from build123d import *

# Parameters (mm, degrees)
SKETCH_1_W               = 60
SKETCH_1_H               = 32
EXTRUDE_1_DEPTH          = 3
SKETCH_3_R               = 36.5
EXTRUDE_2_DEPTH          = 2
SKETCH_4_R               = 1
CUT_EXTRUDE_2_DEPTH      = 10
PATTERN_CIRCULAR_1_COUNT = 8
SKETCH_5_R               = 5
CUT_EXTRUDE_3_DEPTH      = 3
SKETCH_6_R               = 3
EXTRUDE_3_DEPTH          = 5
SKETCH_7_R               = 1.62
CUT_EXTRUDE_4_DEPTH      = 5
SKETCH_9_R               = 2.6
CUT_EXTRUDE_5_DEPTH      = 2
SKETCH_10_R              = 20
EXTRUDE_4_DEPTH          = 3
SKETCH_11_R              = 1.25
CUT_EXTRUDE_6_DEPTH      = 10
PATTERN_CIRCULAR_2_COUNT = 4
SKETCH_12_W              = 42.513020476
SKETCH_12_H              = 32
CUT_EXTRUDE_7_DEPTH      = 3
SKETCH_13_R              = 6
CUT_EXTRUDE_8_DEPTH      = 10


with BuildPart() as part:
    # 草图1 → 凸台-拉伸1 (new body)
    with BuildSketch(Plane.XY):
        with Locations((-44.89426993, 6.0842078)):
            Rectangle(SKETCH_1_W, SKETCH_1_H)
    extrude(amount=EXTRUDE_1_DEPTH)

    # 草图3 → 凸台-拉伸2 (add)
    with BuildSketch(Plane.XY.offset(3)):
        with Locations((-44.89426993, 6.0842078)):
            Circle(SKETCH_3_R)
    extrude(amount=EXTRUDE_2_DEPTH)

    # 草图4 → 切除-拉伸2 (cut)
    with BuildSketch(Plane.XY.offset(5)):
        with Locations((-44.89426993, 29.0842078)):
            Circle(SKETCH_4_R)
    cut_extrude_2 = extrude(amount=-CUT_EXTRUDE_2_DEPTH, mode=Mode.SUBTRACT)

    # 阵列(圆周)1: 切除-拉伸2 ×8 about axis
    pattern_circular_1_axis = Axis((-44.89426993, 6.0842078, 0), (0, 0, 1))
    for i in range(1, PATTERN_CIRCULAR_1_COUNT):
        add(cut_extrude_2.rotate(pattern_circular_1_axis, i * 360 / PATTERN_CIRCULAR_1_COUNT), mode=Mode.SUBTRACT)

    # 草图5 → 切除-拉伸3 (cut)
    with BuildSketch(Plane(origin=(0, 0, 0), x_dir=(-1, 0, 0), z_dir=(0, 0, -1))):
        with Locations((28.630813963, 22.347663767)):
            Circle(SKETCH_5_R)
        with Locations((61.157725897, 22.347663767)):
            Circle(SKETCH_5_R)
        with Locations((28.630813963, -10.179248167)):
            Circle(SKETCH_5_R)
        with Locations((61.157725897, -10.179248167)):
            Circle(SKETCH_5_R)
    extrude(amount=-CUT_EXTRUDE_3_DEPTH, mode=Mode.SUBTRACT)

    # 草图6 → 凸台-拉伸3 (add)
    with BuildSketch(Plane(origin=(0, 0, 0), x_dir=(-1, 0, 0), z_dir=(0, 0, -1))):
        with Locations((21.89426993, 6.0842078)):
            Circle(SKETCH_6_R)
        with Locations((67.89426993, 6.0842078)):
            Circle(SKETCH_6_R)
    extrude(amount=-EXTRUDE_3_DEPTH)

    # 草图7 → 切除-拉伸4 (cut)
    with BuildSketch(Plane(origin=(0, 0, 0), x_dir=(-1, 0, 0), z_dir=(0, 0, -1))):
        with Locations((19.89426993, 12.0842078)):
            Circle(SKETCH_7_R)
        with Locations((19.89426993, 0.0842078)):
            Circle(SKETCH_7_R)
        with Locations((69.89426993, 12.0842078)):
            Circle(SKETCH_7_R)
        with Locations((69.89426993, 0.0842078)):
            Circle(SKETCH_7_R)
    extrude(amount=-CUT_EXTRUDE_4_DEPTH, mode=Mode.SUBTRACT)

    # 草图9 → 切除-拉伸5 (cut)
    with BuildSketch(Plane.XY.offset(5)):
        with Locations((-69.89426993, 12.0842078)):
            Circle(SKETCH_9_R)
        with Locations((-69.89426993, 0.0842078)):
            Circle(SKETCH_9_R)
        with Locations((-19.89426993, 12.0842078)):
            Circle(SKETCH_9_R)
        with Locations((-19.89426993, 0.0842078)):
            Circle(SKETCH_9_R)
    extrude(amount=-CUT_EXTRUDE_5_DEPTH, mode=Mode.SUBTRACT)

    # 草图10 → 凸台-拉伸4 (add)
    with BuildSketch(Plane.XY.offset(5)):
        with Locations((-44.89426993, 6.0842078)):
            Circle(SKETCH_10_R)
    extrude(amount=EXTRUDE_4_DEPTH)

    # 草图11 → 切除-拉伸6 (cut)
    with BuildSketch(Plane.XY.offset(8)):
        with Locations((-44.89426993, 14.0842078)):
            Circle(SKETCH_11_R)
    cut_extrude_6 = extrude(amount=-CUT_EXTRUDE_6_DEPTH, mode=Mode.SUBTRACT)

    # 阵列(圆周)2: 切除-拉伸6 ×4 about axis
    pattern_circular_2_axis = Axis((-44.89426993, 6.0842078, 0), (0, 0, 1))
    for i in range(1, PATTERN_CIRCULAR_2_COUNT):
        add(cut_extrude_6.rotate(pattern_circular_2_axis, i * 360 / PATTERN_CIRCULAR_2_COUNT), mode=Mode.SUBTRACT)

    # 草图12 → 切除-拉伸7 (cut)
    with BuildSketch(Plane(origin=(0, 0, 0), x_dir=(-1, 0, 0), z_dir=(0, 0, -1))):
        with Locations((44.89426993, 6.0842078)):
            Rectangle(SKETCH_12_W, SKETCH_12_H)
    extrude(amount=-CUT_EXTRUDE_7_DEPTH, mode=Mode.SUBTRACT)

    # 草图13 → 切除-拉伸8 (cut)
    with BuildSketch(Plane.XY.offset(8)):
        with Locations((-44.89426993, 6.0842078)):
            Circle(SKETCH_13_R)
    extrude(amount=-CUT_EXTRUDE_8_DEPTH, mode=Mode.SUBTRACT)


solid = part.part
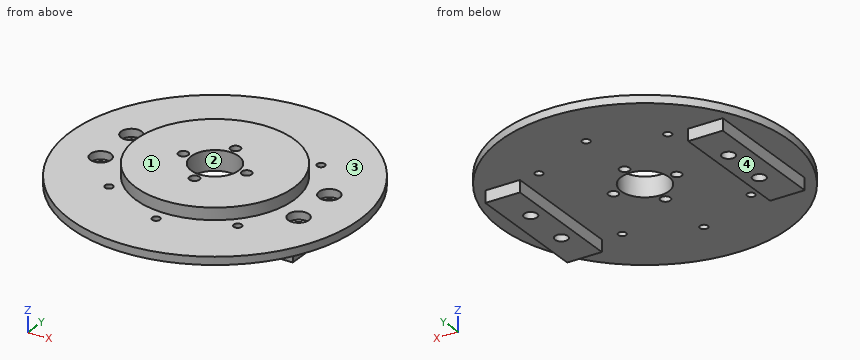
The model under review builds one solid part; all positions refer to its coordinate system, in mm. Face numbers are marked on the shaded views. A direction names the side the tool comes from. Round coordinates to 2 decimals unless told otherwise and drop trailing zeros. Order: outer loops, then holes, each group sorted by start corner. A loop starts at its lowest first (then second) coordinate and runs counter-clockwise, first axis right, second up. Notation, with made-up numbers: (58.25, 48.5) -> (78.25, 48.5) arc R15 ccw to (78.25, 68.5) -> close; hole circle Ø4 at (11.5, 59.25). An arc over 180 degrees is marked (long way). Return JSON: item names as keys, results as strings.
1. Take a section at B-B (x = -20). Write out the cut boundary in (y, z), then the cut area to 3 significant figures.
Answer block:
{"outline": "(-20.61, 3) -> (-9.92, 3) -> (-9.92, 0) -> (-1.53, 0) -> (-1.53, 3) -> (-2.51, 3) -> (-2.51, 5) -> (-20.61, 5) -> close; (1.7, 0) -> (10.47, 0) -> (10.47, 3) -> (9.49, 3) -> (9.49, 5) -> (2.68, 5) -> (2.68, 3) -> (1.7, 3) -> close; (13.7, 0) -> (22.08, 0) -> (22.08, 3) -> (32.78, 3) -> (32.78, 5) -> (14.68, 5) -> (14.68, 3) -> (13.7, 3) -> close", "area": "163 mm²"}
2. Take a section at D-D (y = -4). Write out the cut boundary in (x, z).
Answer block:
{"outline": "(-79.97, 3) -> (-74.89, 3) -> (-74.89, 0) -> (-66.15, 0) -> (-66.15, 3) -> (-23.64, 3) -> (-23.64, 0) -> (-14.89, 0) -> (-14.89, 3) -> (-9.81, 3) -> (-9.81, 5) -> (-27.62, 5) -> (-27.62, 8) -> (-62.17, 8) -> (-62.17, 5) -> (-79.97, 5) -> close"}
3. For L1, parallel to X at y = -2, z = 2; L2, parallel to Z at x = -33, y = 10.5; L3, parallel to Z at x = -65, y = 33.5, list the stretches that pass through material, from the lowest coordinate up. Write a range as [from, to].
Answer block:
{"L1": "x = [-74.89, -66.15], [-23.64, -14.89]", "L2": "z = [3, 8]", "L3": "z = [3, 5]"}
4. Take a section at C-C (x = -48). Write out the cut boundary in (y, z), then the cut area to 3 significant figures.
Answer block:
{"outline": "(-30.28, 3) -> (0.95, 3) -> (0.95, 8) -> (-13.67, 8) -> (-13.67, 5) -> (-30.28, 5) -> close; (11.22, 3) -> (42.45, 3) -> (42.45, 5) -> (25.84, 5) -> (25.84, 8) -> (11.22, 8) -> close", "area": "213 mm²"}
5. Insertion check: P1, Ø3, axis at x = -19.89, y = 0.08, coming from the -Z side; P2, Ø3.5, axis at x = -69, z = 2, coming from the -Y side; P3, Ø1.5, axis at x = -59.5, z = 4, coming from the +Y side; P4, Ø1.5, axis at y = 10.5, z = 3.5, coming from the -X side. Each pin has a flat end and moves straight along its axis. Give the tip position at first contact, or say it passes through.
Answer block:
{"P1": "passes through", "P2": "stops at y = -22.52", "P3": "stops at y = 39.85", "P4": "stops at x = -81.21"}
6. For the marked faces 3 and 4, list the 3-axis set-ups (+Z, -Z, +X, -X, +Y, -Y) from which the entire face can be reached by the end or side of a thin tool; tool diameter is ignored.
Answer block:
{"face 3": "+Z", "face 4": "-Z, +X, -X, +Y, -Y"}
7. The part is to be moulded in two halves that separate along Y. For the marked faces 1 and 2, say which applies: +Y half, -Y half, draft (parallel to the pull), parting line (faces both ways), or undercut.
Answer block:
{"face 1": "draft", "face 2": "undercut"}
8. Take a section at A-A (z = 1). Write out the cut boundary in (x, y).
Answer block:
{"outline": "(-74.89, -9.92) -> (-66.15, -9.92) -> (-66.15, 22.08) -> (-74.89, 22.08) -> close; (-23.64, -9.92) -> (-14.89, -9.92) -> (-14.89, 22.08) -> (-23.64, 22.08) -> close; hole circle Ø3.24 at (-69.89, 0.08); hole circle Ø3.24 at (-69.89, 12.08); hole circle Ø3.24 at (-19.89, 0.08); hole circle Ø3.24 at (-19.89, 12.08)"}
